Verification items for the finished model (mm, model axes). Face numbers are marked on the shaded views. A direction names the side the tool comes from. Coordinates: 2 decimals unless noted, no trailing zeros. Order: outer loops, then holes, each group sorted by start corner. A loop starts at its lowest first (then second) coordinate and runs counter-clockwise, first axis right, second up. Notation, with made-up numbers: M -7.5,72 L 29.5,72 A11 ccw 29.5,80 Z; hole C -17.5,6 d6. An arc over 180 degrees is marked long. Return JSON: item names as keys, results as strings. Group by question number.
Q1. Mould release check, pull along X, two halves, no side actions. Record for the marked faces 3, 4 and 5: pulls with the +X half, pulls with the -X half, needs draft (parallel to the pull), parting line crosses it, or undercut.
Q2. Access from +Z, -Z, +X, -X, +Y, -Y to the whole of each face (thin tool, end or side, straight path). Record for the marked faces 1 and 2.
Q3. Go/stop test with flat-tipped pins: pin 1 Ø1.5 at (y, z) = (0, -2.5) entering from -X; pin 2 Ø4.5 at (y, z) = (0, 0) entering from +X. Record where each tip stops, or that it passes through.
Q4. Section check A-A, the plane x = 0. Enter the section's corners in (y, z).
Q5. Section check C-C, the plane x = 19. Enter the section's corners in (y, z), then the cut area to 3 significant figures.
Q6. Section check D-D, the plane y = -1.75. Count the separate pieces of the cut face and the enclosed holes in it, then the cut area to 3 significant figures.
Q7. Thickness scan on probe 1 along X at (y, z) = (0, -4.5); probe 2 along Z at (x, y) = (12.1, 0); probe 3 along Z at (x, y) = (10, -4). Record the ranges inside material, lowest first.
Q8. Section check B-B, the plane x = 8.5. Enter the section's corners in (y, z), then the cut area to 3 significant figures.
Autodesk Inventor part; units mm, degrees
ref_plane "th1_XY" through (23.8252, 3.175, 0) normal (0, 0, 1) x (1, 0, 0)
ref_plane "th1_YZ" through (23.8252, 3.175, 0) normal (1, 0, 0) x (0, 1, 0)
ref_plane "th1_ZX" through (23.8252, 3.175, 0) normal (0, 1, 0) x (0, 0, 1)
sketch "Sketch_1" plane through (0, 0, 0) normal (0, 0, 1) x (1, 0, 0)
  line L0 (-6.35, 6.35) -> (-6.35, -6.35)
  line L1 (-6.35, -6.35) -> (23.8252, -6.35)
  line L2 (23.8252, -6.35) -> (23.8252, 6.35)
  line L3 (23.8252, 6.35) -> (-6.35, 6.35)
extrude "Extrusion1" add sketch "Sketch_1" along normal mid plane 12.7
sketch "Sketch_2" plane through (0, 0, 0) normal (0, 1, 0) x (-1, 0, 0)
  line L0 (6.35, -3.3338) -> (6.35, 3.3338)
  line L1 (6.35, 3.3338) -> (-11.1252, 3.3338)
  line L2 (-11.1252, 3.3338) -> (-11.1252, -3.3338)
  line L3 (-11.1252, -3.3338) -> (6.35, -3.3338)
extrude "Extrusion2" cut sketch "Sketch_2" along normal mid plane 12.7
sketch "Sketch3" plane through (23.8252, -6.35, 6.35) normal (1, 0, 0) x (0, 0, -1)
  point P0 (6.35, 6.35)
hole "Drilling 1" at (23.8252, 0, 0) direction (-1, 0, 0) diameter 5.3594 depth 11.176 countersink diameter 6.35 countersink angle 90
sketch "Sketch4" plane through (12.6492, 0, 0) normal (1, 0, 0) x (0, 0, -1)
  point P0 (0, 0)
hole "Drilling 2" at (12.6492, 0, 0) direction (-1, 0, 0) diameter 5.4102 depth 1.524
sketch "Sketch_5" plane through (0, 0, 0) normal (1, 0, 0) x (0, 1, 0)
  line L0 (0, -6.35) -> (0, 6.35)
  line L1 (0, 6.35) -> (4.337, 6.35)
  line L2 (4.337, 6.35) -> (3.194, 5.207)
  line L3 (3.194, 5.207) -> (3.194, -5.207)
  line L4 (3.194, -5.207) -> (4.337, -6.35)
  line L5 (4.337, -6.35) -> (0, -6.35)
  line L6 (0, -6.35) -> (0, 6.35)
revolve "Revolution1" cut sketch "Sketch_5" angle 360 about axis through (0, 0, -6.35) along (0, 0, -1)
sketch "Sketch_9" plane through (0, 0, 0) normal (0, 0, 1) x (1, 0, 0)
  line L0 (30.1752, 0) -> (23.8252, 0)
  line L1 (23.8252, 0) -> (23.8252, 6.35)
  arc A0 (23.8252, 6.35) -> (21.2852, 12.7) centre (6.6802, 3.175) ccw
  line L2 (21.2852, 12.7) -> (30.1752, 12.7)
  line L3 (30.1752, 12.7) -> (30.1752, 0)
  line L4 (30.1752, 0) -> (23.8252, 0)
revolve "Revolution2" cut sketch "Sketch_9" angle 360 about axis through (30.1752, 0, 0) along (1, 0, 0)
sketch "Sketch_10" plane through (0, 0, 0) normal (0, 0, 1) x (1, 0, 0)
  line L0 (-6.35, 0) -> (-12.7, 0)
  line L1 (-12.7, 0) -> (-12.7, 12.7)
  line L2 (-12.7, 12.7) -> (-3.81, 12.7)
  arc A0 (-3.81, 12.7) -> (-6.35, 6.35) centre (10.795, 3.175) ccw
  line L3 (-6.35, 6.35) -> (-6.35, 0)
  line L4 (-6.35, 0) -> (-12.7, 0)
revolve "Revolution3" cut sketch "Sketch_10" angle 360 about axis through (-6.35, 0, 0) along (1, 0, 0)
ref_plane "th1_XY" through (23.8252, 3.175, 0) normal (0, 0, 1) x (1, 0, 0)
ref_plane "th1_YZ" through (23.8252, 3.175, 0) normal (1, 0, 0) x (0, 1, 0)
ref_plane "th1_ZX" through (23.8252, 3.175, 0) normal (0, 1, 0) x (0, 0, 1)
ref_plane "th2_XY" through (23.8252, -3.175, 0) normal (0, 0, 1) x (1, 0, 0)
ref_plane "th2_YZ" through (23.8252, -3.175, 0) normal (1, 0, 0) x (0, 1, 0)
ref_plane "th2_ZX" through (23.8252, -3.175, 0) normal (0, 1, 0) x (0, 0, 1)
ref_plane "rod_clevis_body_XY" through (0, 0, 0) normal (0, 0, 1) x (1, 0, 0)
ref_plane "rod_clevis_body_YZ" through (0, 0, 0) normal (1, 0, 0) x (0, 1, 0)
ref_plane "rod_clevis_body_ZX" through (0, 0, 0) normal (0, 1, 0) x (0, 0, 1)
ref_plane "piston_rod_clevis_XY" through (23.8252, 0, 0) normal (1, 0, 0) x (0, 0, -1)
ref_plane "piston_rod_clevis_YZ" through (23.8252, 0, 0) normal (0, 0, -1) x (0, 1, 0)
ref_plane "piston_rod_clevis_ZX" through (23.8252, 0, 0) normal (0, 1, 0) x (1, 0, 0)
ref_plane "dummy_XY" through (0, 0, 0) normal (0, 0, 1) x (1, 0, 0)
ref_plane "dummy_YZ" through (0, 0, 0) normal (1, 0, 0) x (0, 1, 0)
ref_plane "dummy_ZX" through (0, 0, 0) normal (0, 1, 0) x (0, 0, 1)
ref_plane "l11_XY" through (23.8252, 6.35, 0) normal (0, 0, 1) x (1, 0, 0)
ref_plane "l11_YZ" through (23.8252, 6.35, 0) normal (1, 0, 0) x (0, 1, 0)
ref_plane "l11_ZX" through (23.8252, 6.35, 0) normal (0, 1, 0) x (0, 0, 1)
ref_plane "l12_XY" through (0, 6.35, 0) normal (0, 0, 1) x (1, 0, 0)
ref_plane "l12_YZ" through (0, 6.35, 0) normal (1, 0, 0) x (0, 1, 0)
ref_plane "l12_ZX" through (0, 6.35, 0) normal (0, 1, 0) x (0, 0, 1)
ref_plane "l1_XY" through (23.8252, 6.35, 0) normal (0, 0, 1) x (1, 0, 0)
ref_plane "l1_YZ" through (23.8252, 6.35, 0) normal (1, 0, 0) x (0, 1, 0)
ref_plane "l1_ZX" through (23.8252, 6.35, 0) normal (0, 1, 0) x (0, 0, 1)
ref_plane "h1_XY" through (-6.35, 6.35, 0) normal (0, 0, 1) x (1, 0, 0)
ref_plane "h1_YZ" through (-6.35, 6.35, 0) normal (1, 0, 0) x (0, 1, 0)
ref_plane "h1_ZX" through (-6.35, 6.35, 0) normal (0, 1, 0) x (0, 0, 1)
ref_plane "l2_XY" through (-6.35, 6.35, 0) normal (0, 0, 1) x (1, 0, 0)
ref_plane "l2_YZ" through (-6.35, 6.35, 0) normal (1, 0, 0) x (0, 1, 0)
ref_plane "l2_ZX" through (-6.35, 6.35, 0) normal (0, 1, 0) x (0, 0, 1)
ref_plane "h2_XY" through (-6.35, -6.35, 0) normal (0, 0, 1) x (1, 0, 0)
ref_plane "h2_YZ" through (-6.35, -6.35, 0) normal (1, 0, 0) x (0, 1, 0)
ref_plane "h2_ZX" through (-6.35, -6.35, 0) normal (0, 1, 0) x (0, 0, 1)
ref_plane "w11_XY" through (-6.35, 0, -3.3338) normal (0, 1, 0) x (1, 0, 0)
ref_plane "w11_YZ" through (-6.35, 0, -3.3338) normal (1, 0, 0) x (0, 0, -1)
ref_plane "w11_ZX" through (-6.35, 0, -3.3338) normal (0, 0, -1) x (0, 1, 0)
ref_plane "w12_XY" through (-6.35, 0, 3.3338) normal (0, 1, 0) x (1, 0, 0)
ref_plane "w12_YZ" through (-6.35, 0, 3.3338) normal (1, 0, 0) x (0, 0, -1)
ref_plane "w12_ZX" through (-6.35, 0, 3.3338) normal (0, 0, -1) x (0, 1, 0)
ref_plane "l21_XY" through (23.8252, 0, 0) normal (0, 1, 0) x (1, 0, 0)
ref_plane "l21_YZ" through (23.8252, 0, 0) normal (1, 0, 0) x (0, 0, -1)
ref_plane "l21_ZX" through (23.8252, 0, 0) normal (0, 0, -1) x (0, 1, 0)
ref_plane "l22_XY" through (11.1252, 0, 0) normal (0, 1, 0) x (1, 0, 0)
ref_plane "l22_YZ" through (11.1252, 0, 0) normal (1, 0, 0) x (0, 0, -1)
ref_plane "l22_ZX" through (11.1252, 0, 0) normal (0, 0, -1) x (0, 1, 0)
ref_plane "w1_XY" through (23.8252, 0, -6.35) normal (0, 1, 0) x (1, 0, 0)
ref_plane "w1_YZ" through (23.8252, 0, -6.35) normal (1, 0, 0) x (0, 0, -1)
ref_plane "w1_ZX" through (23.8252, 0, -6.35) normal (0, 0, -1) x (0, 1, 0)
ref_plane "w2_XY" through (23.8252, 0, 6.35) normal (0, 1, 0) x (1, 0, 0)
ref_plane "w2_YZ" through (23.8252, 0, 6.35) normal (1, 0, 0) x (0, 0, -1)
ref_plane "w2_ZX" through (23.8252, 0, 6.35) normal (0, 0, -1) x (0, 1, 0)
ref_plane "to_cylinder_XY" through (11.1252, 0, 0) normal (1, 0, 0) x (0, 0, -1)
ref_plane "to_cylinder_YZ" through (11.1252, 0, 0) normal (0, 0, -1) x (0, 1, 0)
ref_plane "to_cylinder_ZX" through (11.1252, 0, 0) normal (0, 1, 0) x (1, 0, 0)
properties part number "D-14055"
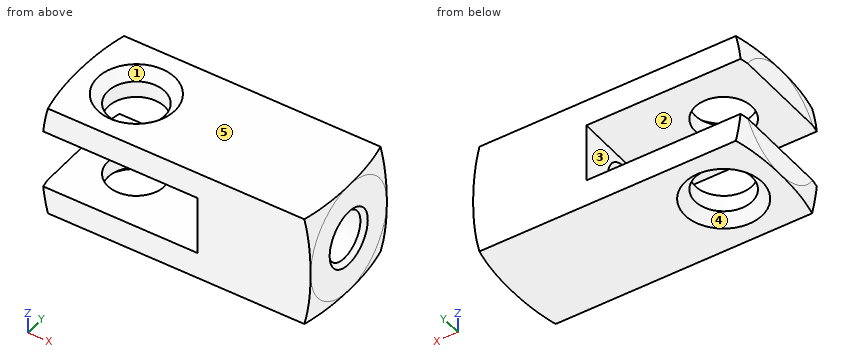
Numbers:
{
 "1": {"face 3": "pulls with the -X half", "face 4": "undercut", "face 5": "needs draft"},
 "2": {"face 1": "+Z", "face 2": "-X, +Y, -Y"},
 "3": {"pin 1": "stops at x = 11.13", "pin 2": "passes through"},
 "4": {"outline": "M -6.35,-6.35 L -4.34,-6.35 L -3.19,-5.21 L -3.19,-3.33 L -6.35,-3.33 Z; M -6.35,3.33 L -3.19,3.33 L -3.19,5.21 L -4.34,6.35 L -6.35,6.35 Z; M 3.19,-5.21 L 4.34,-6.35 L 6.35,-6.35 L 6.35,-3.33 L 3.19,-3.33 Z; M 3.19,3.33 L 6.35,3.33 L 6.35,6.35 L 4.34,6.35 L 3.19,5.21 Z"},
 "5": {"outline": "M -6.35,-6.35 L 6.35,-6.35 L 6.35,6.35 L -6.35,6.35 Z; hole C 0,0 d5.36", "area": "139 mm2"},
 "6": {"separate pieces": "4", "enclosed holes": "0", "area": "179 mm2"},
 "7": {"probe 1": "x = -6.35 to -3.19, 3.19 to 23.83", "probe 2": "z = -6.35 to -2.71, 2.71 to 6.35", "probe 3": "z = -6.35 to -3.33, 3.33 to 6.35"},
 "8": {"outline": "M -6.35,-6.35 L 6.35,-6.35 L 6.35,-3.33 L -6.35,-3.33 Z; M -6.35,3.33 L 6.35,3.33 L 6.35,6.35 L -6.35,6.35 Z", "area": "76.6 mm2"}
}
